Here's the drawing with two shaded views (mm, measured from the low corner). I have some questions. A direction names the side the tool comes from. Give positions to 0.01 mm unless a question says otherwise; leave off trailing zeros. Loops run counter-clockwise (first coordinate to the right, second up) from the corner with the lowest first, then second, coordinate; pieces in that order, holes last. Notation, with made-up numbers: (73.25, 7.25) - (94.25, 7.25) arc R29 cw to (94.25, 31.25) - close; hole circle Ø11 at (41.25, -19). An arc over 180 degrees is marked (long way). Use one line per item in the form item = value.
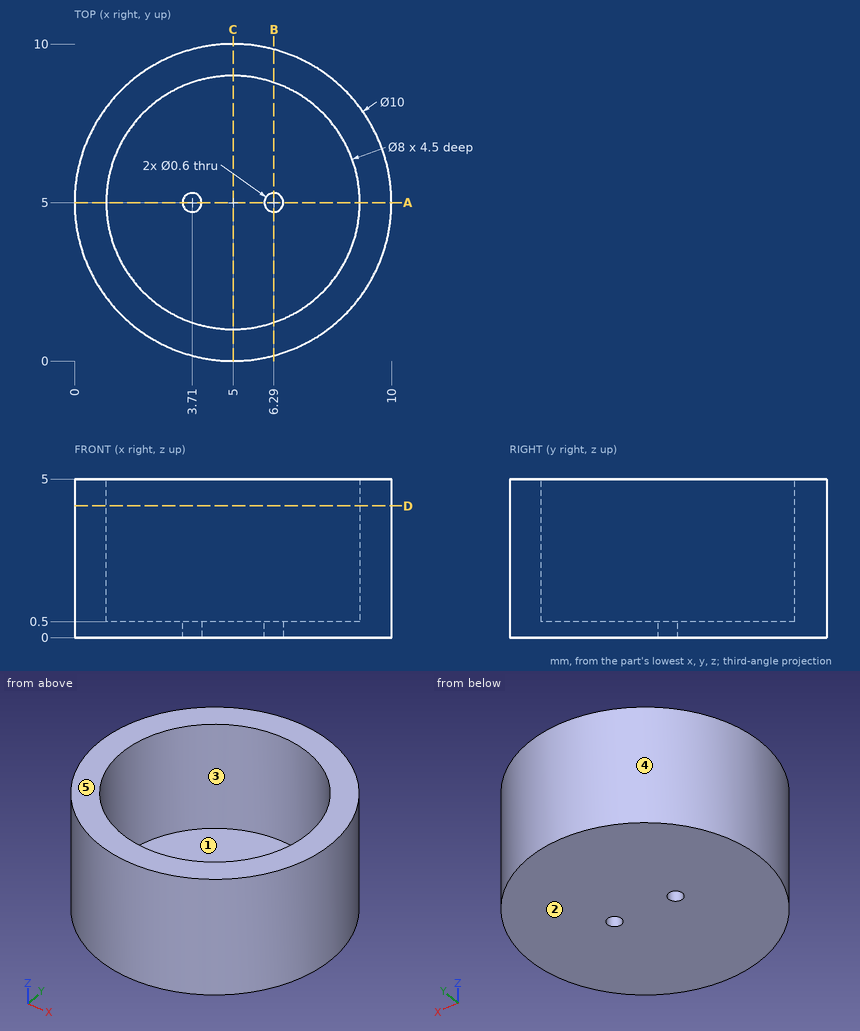
(1) If we section it at C-C (x = 5): List the corners of the cut face in (y, z) for me.
Geometry says:
outline = (0, 0) - (10, 0) - (10, 5) - (9, 5) - (9, 0.5) - (1, 0.5) - (1, 5) - (0, 5) - close
(2) For P1, Ø6, axis at x = 6, y = 9, coming from the -Z side; P2, Ø1, axis at x = 1.5, z = 3.5, coming from the +Y side, each with a flat end and sliding along its axis, tell me the tip position at first contact or that it passes through.
Geometry says:
P1 = 0
P2 = 9
(3) If we section it at B-B (x = 6.29): List the corners of the cut face in (y, z) for me, plus the area to 3 significant figures.
Geometry says:
outline = (0.17, 0) - (4.7, 0) - (4.7, 0.5) - (1.21, 0.5) - (1.21, 5) - (0.17, 5) - close; (5.3, 0) - (9.83, 0) - (9.83, 5) - (8.79, 5) - (8.79, 0.5) - (5.3, 0.5) - close
area = 13.9 mm²
(4) Thinking about a two-plate mould opening in Y: for the marked faces 3, 4 and 5, which applies, pulls with the +Y half, pulls with the -Y half, needs draft (parallel to the pull), parting line crosses it, or undercut?
Geometry says:
face_3 = undercut
face_4 = parting line crosses it
face_5 = needs draft
(5) If we section it at A-A (y = 5): List the corners of the cut face in (x, z) for me, plus the area to 3 significant figures.
Geometry says:
outline = (0, 0) - (3.41, 0) - (3.41, 0.5) - (1, 0.5) - (1, 5) - (0, 5) - close; (4.01, 0) - (5.99, 0) - (5.99, 0.5) - (4.01, 0.5) - close; (6.59, 0) - (10, 0) - (10, 5) - (9, 5) - (9, 0.5) - (6.59, 0.5) - close
area = 13.4 mm²
(6) If we section it at D-D (z = 4.15): List the corners of the cut face in (x, y) for me.
Geometry says:
outline = circle Ø10 at (5, 5); hole circle Ø8 at (5, 5)
(7) If I drill on probe 1 along Y at (x, z) = (5, 2.7); probe 2 along Z at (x, y) = (2.25, 3.75); probe 3 along Y at (x, z) = (3.71, 0.1), over which ranges is the centre line in solid material (lowest first)?
Geometry says:
probe_1 = 0 to 1, 9 to 10
probe_2 = 0 to 0.5
probe_3 = 0.17 to 4.7, 5.3 to 9.83
(8) For the marked faces 1 and 2, which set-ups out of +Z, -Z, +X, -X, +Y, -Y let a thin tool reach every point of the face, with its end or its side?
Geometry says:
face_1 = +Z
face_2 = -Z, +X, -X, +Y, -Y
